Design review of the part built by this model. Coordinates are the model's own, in mm. A direction names the side the tool comes from. Round coordinates to 2 decimals unless told otherwise and drop trailing zeros. Order: outer loops, then holes, each group sorted by start corner. A loop starts at its lowest first (then second) coordinate and runs counter-clockwise, first axis right, second up. Notation, with made-up numbers: (81, 50.25) - (137, 50.25) arc R21 ccw to (137, 62.25) - close; hole circle Ø10 at (84, -27). An arc over 180 degrees is marked (long way). Use CSV: the item, a comma, the result in double quotes. Start each with the question number.
Autodesk Inventor part; units mm, degrees
ref_plane "YZ Plane" through (0, 0, 0) normal (1, 0, 0) x (0, 1, 0)
ref_plane "XZ Plane" through (0, 0, 0) normal (0, 1, 0) x (-1, 0, 0)
ref_plane "XY Plane" through (0, 0, 0) normal (0, 0, 1) x (1, 0, 0)
sketch "Sketch1" plane through (0, 0, 0) normal (0, 1, 0) x (-1, 0, 0)
  line L0 (7, -2.85) -> (-7, -2.85)
  line L1 (-7, -2.85) -> (-7, 2.85)
  line L2 (-7, 2.85) -> (7, 2.85)
  line L3 (7, 2.85) -> (7, -2.85)
  line L4 (7, -2.85) -> (-7, 2.85) construction
  line L5 (-7, -2.85) -> (7, 2.85) construction
  point P0 (0, 0)
  dimension "d0" = 14
  dimension "d1" = 5.7
extrude "Extrusion1" add sketch "Sketch1" along normal blind 2
sketch "Sketch2" plane through (0, 2, 0) normal (0, 1, 0) x (1, 0, 0)
  line L0 (7, 2.85) -> (-7, 2.85)
  line L1 (-7, -2.85) -> (7, -2.85)
  line L2 (-7, 2.85) -> (-5, 2.85)
  line L3 (-5, 2.85) -> (-5, -2.85)
  line L4 (-5, -2.85) -> (-7, -2.85)
  line L5 (-7, -2.85) -> (-7, 2.85)
  line L6 (-9.8, 0) -> (9.8, 0)
  line L7 (0, 3.99) -> (0, -3.99)
  line L8 (7, 2.85) -> (5, 2.85)
  line L9 (5, 2.85) -> (5, -2.85)
  line L10 (5, -2.85) -> (7, -2.85)
  line L11 (7, -2.85) -> (7, 2.85)
  point P0 (0, 0)
  dimension "d4" = 2
extrude "Extrusion2" add sketch "Sketch2" along normal blind 4 contours L11 L6 L9 L0 | L11 L1 L9 L6 | L3 L6 L5 L0 | L3 L1 L5 L6
equation "\"BendRadius\" = Thickness"
equation "\"BendReliefWidth\" = Thickness"
equation "\"BendReliefDepth\" = 0.5 * Thickness"
equation "\"CornerReliefSize\" = 4 * Thickness"
equation "\"MinimumRemnant\" = 2 * Thickness"
equation "\"TransitionRadius\" = BendRadius"
equation "\"JacobiRadiusSize\" = BendRadius"
equation "\"GapSize\" = Thickness"
properties part number "_3DPrint"
Q1. Take a section at A-A (y = 4.05). State the section outline as (x, z) points, plus the area to 3 significant figures.
Q2. Tool access review of faces 4 (the flat face through (-6, 6, 0)), 5 (the flat face through (0, 2, 0)): name each direction out of +Z, -Z, +X, -X, +Y, -Y from which nothing blocks a thin tool from reaching the whole face with its end or side.
Q3. The part is to be moulded in two halves that separate along X. For faces 1 (the flat face through (-5, 4, 0)), 2 (the flat face through (0, 0, 0)), 3 (the flat face through (7, 3, 0)), say which applies: +X half, -X half, draft (parallel to the pull), parting line (faces both ways), or undercut.
Q4. Take a section at B-B (z = 0.65). State the section outline as (x, y) points, plus the area to 3 significant figures.
Q5. Take a section at C-C (x = -2.75). State the section outline as (y, z) points, plus the area to 3 significant figures.
Q6. For L1, parallel to X at y = 2.85, z = -1.35; L2, parallel to Y at x = -2, z = 2.1, list the stretches that pass through material, from the lowest coordinate up. Write a range as [from, to].
Q7. Clearance check with a flat-ended pin moving along its axis: pin 1 (3 mm diameter, centred on x = 1, z = 0.5, fed in from +Y). State where the tip first meets the part, or that it passes through.
Findings below:
1,outline,"(-7, -2.85) - (-5, -2.85) - (-5, 2.85) - (-7, 2.85) - close; (5, -2.85) - (7, -2.85) - (7, 2.85) - (5, 2.85) - close"
1,area,"22.8 mm^2"
2,face 4,"+Z, -Z, +X, -X, +Y"
2,face 5,"+Z, -Z, +Y"
3,face 1,"undercut"
3,face 2,"draft"
3,face 3,"+X half"
4,outline,"(-7, 0) - (7, 0) - (7, 6) - (5, 6) - (5, 2) - (-5, 2) - (-5, 6) - (-7, 6) - close"
4,area,"44.0 mm^2"
5,outline,"(0, -2.85) - (2, -2.85) - (2, 2.85) - (0, 2.85) - close"
5,area,"11.4 mm^2"
6,L1,"x = [-7, -5], [5, 7]"
6,L2,"y = [0, 2]"
7,pin 1,"stops at y = 2"
